from build123d import *

# Parameters (mm, degrees)
SKETCH_W        = 11
SKETCH_H        = 19
PAD_DEPTH       = 1.5
SKETCH001_R     = 1.75
POCKET_DEPTH    = 1.5
SKETCH002_R     = 3
POCKET001_DEPTH = 0.5
POCKET002_DEPTH = 1.5
FILLET_R        = 5


with BuildPart() as part:
    # Sketch → Pad (new body)
    with BuildSketch(Plane.XY):
        with Locations((0, 1.5)):
            Rectangle(SKETCH_W, SKETCH_H)
    extrude(amount=PAD_DEPTH)

    # Sketch001 (on Face6 of Pad) → Pocket (cut)
    with BuildSketch(Plane.XY.offset(1.5)):
        with Locations((1.5, -3)):
            Circle(SKETCH001_R)
    extrude(amount=-POCKET_DEPTH, mode=Mode.SUBTRACT)

    # Sketch002 (on Face5 of Pocket) → Pocket001 (cut)
    with BuildSketch(Plane.XY.offset(1.5)):
        with Locations((1.5, -3)):
            Circle(SKETCH002_R)
    extrude(amount=-POCKET001_DEPTH, mode=Mode.SUBTRACT)

    # Sketch003 (on Face5 of Pocket001) → Pocket002 (cut)
    with BuildSketch(Plane.XY.offset(1.5)):
        Polygon((-4, 8.5), (-5.5, 7), (-5.5, -1.5), (-4, -3), align=None)
    extrude(amount=-POCKET002_DEPTH, mode=Mode.SUBTRACT)

    # Fillet
    fillet_edges = [part.edges().sort_by_distance(p)[0] for p in [
        (-5.5, -8, 0.75),
    ]]
    fillet(fillet_edges, radius=FILLET_R)


solid = part.part
Verification items for the finished model (mm, model axes). A direction names the side the tool comes from. Coordinates: 2 decimals unless noted, no trailing zeros. Order: outer loops, then holes, each group sorted by start corner. A loop starts at its lowest first (then second) coordinate and runs counter-clockwise, first axis right, second up. Notation, with made-up numbers: M -1.75,-22.75 L 18.25,-22.75 A23 ccw 18.25,2.25 Z; hole C 46,36.25 d8. An arc over 180 degrees is marked long. One line per item, written item: value. Start each with the question number.
Item 1: Mould release check, pull along X, two halves, no side actions. Record for faces 1 (the cylindrical face through (-4.07, -6.5, 0.76)), 2 (the flat face through (-5, -2, 1)), 3 (the flat face through (0, 11, 1)): pulls with the +X half, pulls with the -X half, needs draft (parallel to the pull), parting line crosses it, or undercut.
Item 2: Sectioned sample at D-D on x = 3. Record the cut outline in (y, z), then the cut area to 3 significant figures.
Item 3: Thickness scan on probe 1 along Y at (x, z) = (1.5, 0.7); probe 2 along Y at (x, z) = (1.5, 1.3); probe 3 along X at (y, z) = (4.75, 0.8). Record the ranges inside material, lowest first.
Item 4: Sectioned sample at A-A on x = 1.5. Record the cut outline in (y, z).
Item 5: Depth check by flat-ended pin: P1, Ø3, axis at x = 2.5, y = -4, coming from the +Z side. Enter the tip coordinate at first touch or a pass-through.
Item 6: Sectioned sample at C-C on y = -2.75. Record the cut outline in (x, z).
Item 7: Access from +Z, -Z, +X, -X, +Y, -Y to the whole of each face (thin tool, end or side, straight path). Record for faces 4 (the flat face through (3.5, -3, 1)), 5 (the flat face through (0, 2, 0)), 6 (the flat face through (-4, 3, 1)).
Item 8: Sectioned sample at B-B on z = 0.55. Record the cut outline in (x, y), then the cut area to 3 significant figures.
Calculated:
1. face 1: pulls with the -X half
1. face 2: undercut
1. face 3: needs draft
2. outline: M -8,0 L -3.9,0 L -3.9,1 L -5.6,1 L -5.6,1.5 L -8,1.5 Z; M -2.1,0 L 11,0 L 11,1.5 L -0.4,1.5 L -0.4,1 L -2.1,1 Z
2. area: 24.1 mm^2
3. probe 1: -8 to -4.75, -1.25 to 11
3. probe 2: -8 to -6, 0 to 11
3. probe 3: -4 to 5.5
4. outline: M -8,0 L -4.75,0 L -4.75,1 L -6,1 L -6,1.5 L -8,1.5 Z; M -1.25,0 L 11,0 L 11,1.5 L 0,1.5 L 0,1 L -1.25,1 Z
5. P1: z = 1
6. outline: M -5.5,0 L -4.25,0 L -4.25,1.5 L -5.5,1.5 Z; M -4,0 L -0.23,0 L -0.23,1 L -1.49,1 L -1.49,1.5 L -4,1.5 Z; M 3.23,0 L 5.5,0 L 5.5,1.5 L 4.49,1.5 L 4.49,1 L 3.23,1 Z
7. face 4: +Z
7. face 5: -Z, +X, -X, +Y, -Y
7. face 6: +Z, -Z
8. outline: M -5.5,-3 A5 ccw -0.5,-8 L 5.5,-8 L 5.5,11 L -5.5,11 L -5.5,7 L -4,8.5 L -4,-3 L -5.5,-1.5 Z; hole C 1.5,-3 d3.5
8. area: 179 mm^2
